Check sheet for the modelled part. Datum: model origin and axes. Units: mm. A direction names the side the tool comes from. Coordinates: 2 decimals unless noted, no trailing zeros. Order: outer loops, then holes, each group sorted by start corner. A loop starts at its lowest first (then second) coordinate and runs counter-clockwise, first axis right, second up.
from build123d import *

# Parameters (mm, degrees)
SKETCH1_W           = 50
SKETCH1_H           = 21
BOSS_EXTRUDE1_DEPTH = 58
SKETCH3_R           = 7.5
CUT_EXTRUDE1_DEPTH  = 24
CUT_EXTRUDE2_REACH  = 66.025
SKETCH4_R           = 5
CUT_EXTRUDE3_START  = -24
SKETCH5_R           = 7.5
CUT_EXTRUDE3_DEPTH  = 24
CUT_EXTRUDE4_REACH  = 66.025
SKETCH6_R           = 4.5
CUT_EXTRUDE5_REACH  = 68.558
SKETCH8_W           = 10
SKETCH8_H           = 18
BOSS_EXTRUDE3_DEPTH = 20
CUT_EXTRUDE6_DEPTH  = 37.5
CUT_EXTRUDE7_REACH  = 85.75
SKETCH13_R          = 2
SKETCH7_R           = 4.1
CUT_EXTRUDE8_DEPTH  = 15


with BuildPart() as part:
    # Sketch1 → Boss-Extrude1 (new body)
    with BuildSketch(Plane(origin=(0, 0, 0), x_dir=(1, 0, 0), z_dir=(0, 1, 0))):
        Rectangle(SKETCH1_W, SKETCH1_H)
    extrude(amount=BOSS_EXTRUDE1_DEPTH)

    # Sketch3 → Cut-Extrude1 (cut)
    with BuildSketch(Plane(origin=(0, 58, 0), x_dir=(1, 0, 0), z_dir=(0, 1, 0))):
        with Locations(Location((-15, 0, 0), (0, 0, 270))):
            Circle(SKETCH3_R)
    extrude(amount=-CUT_EXTRUDE1_DEPTH, mode=Mode.SUBTRACT)

    # Sketch4 → Cut-Extrude2 (cut, up to next)
    with BuildSketch(Plane(origin=(0, 58, 0), x_dir=(1, 0, 0), z_dir=(0, 1, 0)), mode=Mode.PRIVATE) as cut_extrude2_sk1:
        with Locations(Location((15, 0, 0), (0, 0, 270))):
            Circle(SKETCH4_R)
    cut_extrude2_tool1 = extrude(cut_extrude2_sk1.sketch, amount=-CUT_EXTRUDE2_REACH, mode=Mode.PRIVATE) & part.part
    add(cut_extrude2_tool1.solids().sort_by_distance((15, 58, 0))[0], mode=Mode.SUBTRACT)

    # Sketch5 → Cut-Extrude3 (cut)
    with BuildSketch(Plane.XZ.offset(CUT_EXTRUDE3_START)):
        with Locations(Location((-15, 0, 0), (0, 0, 90))):
            Circle(SKETCH5_R)
    extrude(amount=CUT_EXTRUDE3_DEPTH, mode=Mode.SUBTRACT)

    # Sketch6 → Cut-Extrude4 (cut, up to next)
    with BuildSketch(Plane.XZ, mode=Mode.PRIVATE) as cut_extrude4_sk1:
        with Locations(Location((-15, 0, 0), (0, 0, 270))):
            Circle(SKETCH6_R)
    cut_extrude4_tool1 = extrude(cut_extrude4_sk1.sketch, amount=-CUT_EXTRUDE4_REACH, mode=Mode.PRIVATE) & part.part
    add(cut_extrude4_tool1.solids().sort_by_distance((-15, 0, 0))[0], mode=Mode.SUBTRACT)

    # Sketch8 → Cut-Extrude5 (cut, up to next)
    with BuildSketch(Plane.XY.offset(10.5), mode=Mode.PRIVATE) as cut_extrude5_sk1:
        with Locations((0, 29)):
            Rectangle(SKETCH8_W, SKETCH8_H)
    cut_extrude5_tool1 = extrude(cut_extrude5_sk1.sketch, amount=-CUT_EXTRUDE5_REACH, mode=Mode.PRIVATE) & part.part
    add(cut_extrude5_tool1.solids().sort_by_distance((0, 29, 10.5))[0], mode=Mode.SUBTRACT)

    # Sketch11 → Boss-Extrude3 (add, symmetric)
    with BuildSketch(Plane(origin=(0, 29, 0), x_dir=(0, 0, -1), z_dir=(0, 1, 0))):
        Polygon((40.5, 5.5), (40.5, -5.5), (10.5, -15), (10.5, -25), (44.5, -7.5), (44.5, 7.5), (10.5, 25), (10.5, 15), align=None)
    extrude(amount=BOSS_EXTRUDE3_DEPTH, both=True)

    # Sketch12 → Cut-Extrude6 (cut, symmetric)
    with BuildSketch(Plane.ZY):
        Polygon((-44.5, 38), (-10.5, 49), (-44.5, 49), align=None)
        Polygon((-44.5, 20), (-10.5, 9), (-44.5, 9), align=None)
    extrude(amount=CUT_EXTRUDE6_DEPTH, both=True, mode=Mode.SUBTRACT)

    # Sketch13 → Cut-Extrude7 (cut, up to next)
    with BuildSketch(Plane(origin=(0, 0, -44.5), x_dir=(-1, 0, 0), z_dir=(0, 0, -1)), mode=Mode.PRIVATE) as cut_extrude7_sk1:
        with Locations((0, 29)):
            Circle(SKETCH13_R)
    cut_extrude7_tool1 = extrude(cut_extrude7_sk1.sketch, amount=-CUT_EXTRUDE7_REACH, mode=Mode.PRIVATE) & part.part
    add(cut_extrude7_tool1.solids().sort_by_distance((0, 29, -44.5))[0], mode=Mode.SUBTRACT)

    # Sketch7 → Cut-Extrude8 (cut)
    with BuildSketch(Plane.XY.offset(10.5)):
        with Locations((0, 46)):
            Circle(SKETCH7_R)
        with Locations(Location((0, 12, 0), (0, 0, 180))):
            Circle(SKETCH7_R)
    extrude(amount=-CUT_EXTRUDE8_DEPTH, mode=Mode.SUBTRACT)


solid = part.part
(1) Tool access check on faces 1 (the cylindrical face through (-21.324, 12.168, 4.032)), 2 (the flat face through (-0.1, 31.4, -40.5)), 3 (the flat face through (0, 38, 0)). Record the directions out of +Z, -Z, +X, -X, +Y, -Y that give a thin tool (end or side, any length) a straight path to the whole face; none if there is none.
Filled in:
face 1: -Y
face 2: +Y, -Y
face 3: +Z
(2) Release check for a two-part mould opening along Z. For faces 4 (the flat face through (-6, 29, -10.5)), 5 (the flat face through (-10, 24, 0)), 6 (the flat face through (0, 12, -4.5)), 7 (the flat face through (5, 29, 0)) record: +Z half, -Z half, draft (parallel to the pull), parting line (faces both ways), or undercut.
Filled in:
face 4: undercut
face 5: undercut
face 6: +Z half
face 7: draft
(3) Cross-section at B-B (y = 29). Enter the section's corners in (x, z), and give its area (3 significant figures).
Filled in:
outline: (-25, -10.5) - (-7.5, -44.5) - (-2, -44.5) - (-2, -40.5) - (-5.5, -40.5) - (-15, -10.5) - (-5, -10.5) - (-5, 10.5) - (-25, 10.5) - close; (2, -44.5) - (7.5, -44.5) - (25, -10.5) - (25, 10.5) - (5, 10.5) - (5, -10.5) - (15, -10.5) - (5.5, -40.5) - (2, -40.5) - close; hole circle Ø9 at (-15, 0); hole circle Ø10 at (15, 0)
area: 1,170 mm2
(4) Cross-section at D-D (y = 22). Enter the section's corners in (x, z).
Filled in:
outline: (-25, -10.5) - (-7.5, -44.5) - (7.5, -44.5) - (25, -10.5) - (25, 10.5) - (5, 10.5) - (5, -10.5) - (15, -10.5) - (5.5, -40.5) - (-5.5, -40.5) - (-15, -10.5) - (-5, -10.5) - (-5, 10.5) - (-25, 10.5) - close; hole circle Ø15 at (-15, 0); hole circle Ø10 at (15, 0)
(5) Cross-section at A-A (z = 0). Enter the section's corners in (x, y).
Filled in:
outline: (-25, 0) - (-22.5, 0) - (-22.5, 24) - (-19.5, 24) - (-19.5, 34) - (-22.5, 34) - (-22.5, 58) - (-25, 58) - close; (-10.5, 24) - (-7.5, 24) - (-7.5, 0) - (10, 0) - (10, 58) - (-7.5, 58) - (-7.5, 34) - (-10.5, 34) - close; (20, 0) - (25, 0) - (25, 58) - (20, 58) - close; hole (-5, 20) - (5, 20) - (5, 38) - (-5, 38) - close; hole circle Ø8.2 at (0, 12); hole circle Ø8.2 at (0, 46)
(6) Go/stop test with flat-tipped pins: P1, Ø10.5, axis at x = 0, y = 12, coming from the -Z side; P2, Ø3, axis at y = 18, z = -26, coming from the -X side; P3, Ø12, axis at x = -15, z = 0, coming from the -Y side. Record where each tip stops, or that it passes through.
Filled in:
P1: stops at z = -10.5
P2: stops at x = -17.79
P3: stops at y = 24
(7) Cross-section at C-C (x = 0). Enter the section's corners in (y, z).
Filled in:
outline: (0, -10.5) - (20, -10.5) - (20, 10.5) - (16.1, 10.5) - (16.1, -4.5) - (7.9, -4.5) - (7.9, 10.5) - (0, 10.5) - close; (18.71, -40.5) - (20, -44.5) - (27, -44.5) - (27, -40.5) - close; (31, -44.5) - (38, -44.5) - (39.29, -40.5) - (31, -40.5) - close; (38, -10.5) - (58, -10.5) - (58, 10.5) - (50.1, 10.5) - (50.1, -4.5) - (41.9, -4.5) - (41.9, 10.5) - (38, 10.5) - close
(8) Thickness scan on probe 1 along Y at (x, z) = (0, 4.5); probe 2 along X at (y, z) = (28.5, 0); probe 3 along Y at (x, z) = (-1.5, -2). Record the ranges inside material, lowest first.
Filled in:
probe 1: y = 0 to 7.9, 16.1 to 20, 38 to 41.9, 50.1 to 58
probe 2: x = -25 to -19.5, -10.5 to -5, 5 to 10, 20 to 25
probe 3: y = 0 to 8.18, 15.82 to 20, 38 to 42.18, 49.82 to 58
